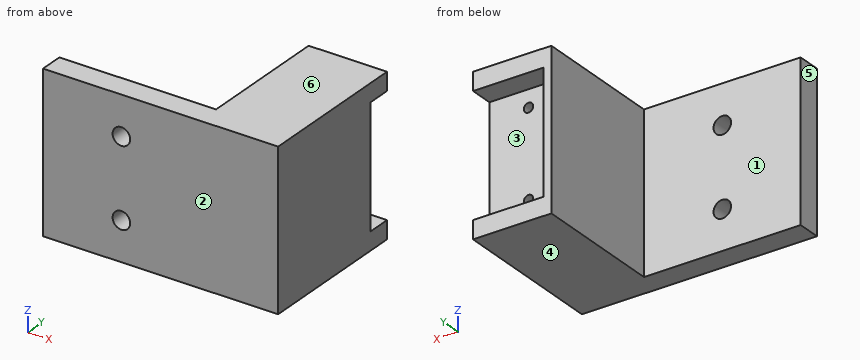
from build123d import *

# Parameters (mm, degrees)
SKETCH1_W                 = 25.4
SKETCH1_H                 = 25.4
BOSS_EXTRUDE1_DEPTH       = 12.7
SKETCH2_W                 = 11.43
SKETCH2_H                 = 19.558
CUT_EXTRUDE1_DEPTH        = 3.81
SHELL2_T                  = -5.08
F_1_64_TAPPED_HOLE2_D     = 1.5113
F_1_64_TAPPED_HOLE2_DEPTH = 6.35
F_1_64_TAPPED_HOLE2_TIP   = 0.454040327
SKETCH12_W                = 38.1
SKETCH12_H                = 25.4
BOSS_EXTRUDE2_DEPTH       = 3.81
SKETCH16_R                = 1.4224
CUT_EXTRUDE2_DEPTH        = 44.994090512


with BuildPart() as part:
    # Sketch1 → Boss-Extrude1 (new body)
    with BuildSketch(Plane(origin=(0, 0, 0), x_dir=(0, 0, -1), z_dir=(1, 0, 0))):
        with Locations((12.7, 12.7)):
            Rectangle(SKETCH1_W, SKETCH1_H)
    extrude(amount=BOSS_EXTRUDE1_DEPTH)

    # Sketch2 → Cut-Extrude1 (cut)
    with BuildSketch(Plane(origin=(0, 25.4, 0), x_dir=(1, 0, 0), z_dir=(0, 1, 0))):
        with Locations((6.985, 12.7)):
            Rectangle(SKETCH2_W, SKETCH2_H)
    extrude(amount=-CUT_EXTRUDE1_DEPTH, mode=Mode.SUBTRACT)

    # Shell2
    shell2_openings = [part.faces().sort_by_distance(p)[0] for p in [
        (6.35, 0, -12.7),
    ]]
    offset(amount=SHELL2_T, openings=shell2_openings, kind=Kind.INTERSECTION)

    # #1-64 Tapped Hole2
    with Locations(Plane(origin=(0, 21.59, 0), x_dir=(1, 0, 0), z_dir=(0, 1, 0))):
        with Locations((6.35, 19.685), (6.35, 5.715)):
            Hole(F_1_64_TAPPED_HOLE2_D / 2, depth=F_1_64_TAPPED_HOLE2_DEPTH)
            with Locations((0, 0, -(F_1_64_TAPPED_HOLE2_DEPTH + F_1_64_TAPPED_HOLE2_TIP / 2))):  # 118° drill point
                Cone(0, F_1_64_TAPPED_HOLE2_D / 2, F_1_64_TAPPED_HOLE2_TIP, mode=Mode.SUBTRACT)

    # Sketch12 → Boss-Extrude2 (add)
    with BuildSketch(Plane.XZ):
        with Locations((-6.35, -12.7)):
            Rectangle(SKETCH12_W, SKETCH12_H)
    extrude(amount=-BOSS_EXTRUDE2_DEPTH)

    # Sketch16 → Cut-Extrude2 (cut, through all)
    with BuildSketch(Plane.XZ):
        with Locations(Location((-12.7, -6.35, 0), (0, 0, 270))):
            Circle(SKETCH16_R)
        with Locations(Location((-12.7, -19.05, 0), (0, 0, 270))):
            Circle(SKETCH16_R)
    extrude(amount=-CUT_EXTRUDE2_DEPTH, mode=Mode.SUBTRACT)


solid = part.part
CAD build for the part. Positions are in the model's coordinates, mm. Face numbers are marked on the shaded views. A direction names the side the tool comes from. Round coordinates to 2 decimals unless told otherwise and drop trailing zeros. Loops run counter-clockwise (first coordinate to the right, second up) from the corner with the lowest first, then second, coordinate; pieces in that order, holes last. Notation, with made-up numbers: M 77.5,21.5 L 116.5,21.5 A18 cw 116.5,56.5 Z; hole C 56.5,58.5 d4. An arc over 180 degrees is marked long. One line per question, with ' | ' between items. Start each with the question number.
Item 1: Wall check: line 1 (Z direction, x = 6.35, y = 19.25); line 2 (X direction, y = 1.4, z = -6.35); line 3 (X direction, y = 5.5, z = -10). Give the ranges that are in metal, low to high.
Item 2: Cut at C-C, the plane z = -11. Write the cut outline in (x, y).
Item 3: Pin check, flat tips, straight feed: pin 1 Ø5 at (x, z) = (-7.5, -20.5) entering from +Y; pin 2 Ø3 at (y, z) = (12, -6.5) entering from -X; pin 3 Ø1.9 at (y, z) = (23, -11.5) entering from +X; pin 4 Ø2.5 at (x, z) = (-12.7, -19.05) entering from +Y. Stop position of each tip, or through.
Item 4: Cut at D-D, the plane y = 13.25. Write the cut outline in (x, z), plus the area to 3 significant figures.
Item 5: Which spindle directions (+Z, -Z, +X, -X, +Y, -Y) get a long thin tool onto all of the face, cutting with end or side? Do the marked faces 1 and 2. Say none if no direction does.
Item 6: Cut at B-B, the plane y = 24. Write the cut outline in (x, z).
Item 7: Cut at A-A, the plane x = -12.7. Write the cut outline in (y, z).
Item 8: Two-plate mould, pull along Z, no slides. Class the marked faces 3, 4, 5 and 6: pulls with the +Z half, pulls with the -Z half, needs draft (parallel to the pull), parting line crosses it, or undercut.
Responses:
1) line 1: z = -25.4 to -20.44, -18.93 to -6.47, -4.96 to 0 | line 2: x = -25.4 to -14.12, -11.28 to 12.7 | line 3: x = 0 to 5.08, 7.62 to 12.7
2) outline: M -25.4,0 L 12.7,0 L 12.7,21.59 L 1.27,21.59 L 1.27,25.4 L 0,25.4 L 0,3.81 L -25.4,3.81 Z; hole M 5.08,3.81 L 7.62,3.81 L 7.62,16.51 L 5.08,16.51 Z
3) pin 1: stops at y = 3.81 | pin 2: stops at x = 0 | pin 3: stops at x = 1.27 | pin 4: passes through
4) outline: M 0,-25.4 L 12.7,-25.4 L 12.7,0 L 0,0 Z; hole M 5.08,-20.32 L 7.62,-20.32 L 7.62,-5.08 L 5.08,-5.08 Z | area: 284 mm²
5) face 1: +Z, -Z, -X, +Y | face 2: +Z, -Z, +X, -X, -Y
6) outline: M 0,-25.4 L 12.7,-25.4 L 12.7,-22.48 L 1.27,-22.48 L 1.27,-2.92 L 12.7,-2.92 L 12.7,0 L 0,0 Z
7) outline: M 0,-25.4 L 3.81,-25.4 L 3.81,-20.47 L 0,-20.47 Z; M 0,-17.63 L 3.81,-17.63 L 3.81,-7.77 L 0,-7.77 Z; M 0,-4.93 L 3.81,-4.93 L 3.81,0 L 0,0 Z
8) face 3: undercut | face 4: pulls with the -Z half | face 5: needs draft | face 6: pulls with the +Z half
